The listing builds one solid part. Answer for the finished solid, in the listing's coordinates (mm). A direction names the side the tool comes from. Coordinates: 2 decimals unless noted, no trailing zeros. Order: outer loops, then holes, each group sorted by start corner. A loop starts at its lowest first (then second) coordinate and runs counter-clockwise, first axis right, second up. Notation, with made-up numbers: (-21.75, 21.5) - (34.25, 21.5) arc R14 ccw to (34.25, 30.5) - close; hole circle Ø4 at (36.5, 16.5). An arc over 180 degrees is marked (long way). Use a Markdown table: item, result. Add a question column.
Item 1: Find the intervals of material crossed by line 1 along X through (y, z) = (0, 11); line 2 along X through (y, z) = (21, -12); line 3 along Z through (x, y) = (17.25, -6), in increasing order.
Item 2: The part is cut by section A-A, the plane z = 0. Give the vertices of the cut face in (x, y), then the cut area to 3 significant figures.
Item 3: The part is cut by section B-B, the plane x = 13.5. Give the vertices of the cut face in (y, z), then the cut area to 3 significant figures.
Item 4: Flat-ended cylindrical pins translate along their axes: P1, Ø1.5, axis at x = 12.5, z = 0.5, coming from the -Y side; P2, Ø1.2, axis at x = 9.5, z = 0.5, coming from the +Y side; P3, Ø2, axis at x = 10.5, y = -6.5, coming from the +Z side. Find the tip coordinate at first contact, or state that the pin passes through.
Item 5: The part is cut by section D-D, the plane x = 6. Give the vertices of the cut face in (y, z), then the cut area to 3 significant figures.
Item 6: For faces 1 (the cylindrical face through (11, 0, 13)), 2 (the cylindrical face through (11, 13, 0)), 3 (the flat face through (9, -7, 2)), 4 (the cylindrical face through (11.59, -0.88, -19.98)), determine the directions among +Z, -Z, +X, -X, +Y, -Y from which every point of the face is accessible in a straight line to the end or side of a thin tool.
Item 7: The part is cut by section C-C, the plane y = -1.5. Give the vertices of the cut face in (x, z).
Item 8: The mould has two halves that part along Z. Classify faces 5 (the flat face through (5, 20.2, 1.9)), 6 (the flat face through (9, -8.1, 0)), 7 (the cylindrical face through (2.535, -18.518, -20.195)): released by +Z, released by -Z, zero draft, split by the parting line, or undercut.
from build123d import *

# Parameters (mm, degrees)
SKETCH_2_R               = 6
CUT_EXTRUDE_1_DEPTH      = 45.55917414
HOLE_WIZARD_M6_1_REACH   = 58.389
HOLE_WIZARD_M6_1_BORE_R  = 2.5
PATTERN_CIRCULAR_1_COUNT = 2
PATTERN_CIRCULAR_1_ANGLE = 90
CUT_EXTRUDE_2_REACH      = 46.559
SKETCH_4_W               = 4
SKETCH_4_H               = 4.2
SKETCH_5_R               = 20
CUT_EXTRUDE_3_DEPTH      = 4


with BuildPart() as part:
    # 草图1 → 旋转1 (revolve)
    with BuildSketch(Plane.XY, mode=Mode.PRIVATE) as revolve_1_sk:
        Polygon((0, 0), (0, 27.4), (5, 27.4), (5, 20), (22, 20), (22, 0), align=None)
    revolve(revolve_1_sk.sketch.rotate(Axis((0, 0, 0), (1, 0, 0)), 90), axis=Axis((0, 0, 0), (1, 0, 0)))

    # 草图2 → 切除-拉伸1 (cut, through all)
    with BuildSketch(Plane.ZY):
        Circle(SKETCH_2_R)
    extrude(amount=-CUT_EXTRUDE_1_DEPTH, mode=Mode.SUBTRACT)

    # M6 螺纹孔1 bore (on position points) → M6 螺纹孔1 (cut, up to next)
    with BuildSketch(Plane(origin=(13.5, 0, 20), x_dir=(1, 0, 0), z_dir=(0, 0, 1)), mode=Mode.PRIVATE) as hole_wizard_m6_1_sk1:
        Circle(HOLE_WIZARD_M6_1_BORE_R)
    hole_wizard_m6_1_tool1 = extrude(hole_wizard_m6_1_sk1.sketch, amount=-HOLE_WIZARD_M6_1_REACH, mode=Mode.PRIVATE) & part.part
    hole_wizard_m6_1 = hole_wizard_m6_1_tool1.solids().sort_by_distance((13.5, 0, 20))[0]
    add(hole_wizard_m6_1, mode=Mode.SUBTRACT)

    # 阵列(圆周)1: M6 螺纹孔1 ×2 about axis
    pattern_circular_1_axis = Axis((22, 0, 0), (-1, 0, 0))
    for i in range(1, PATTERN_CIRCULAR_1_COUNT):
        add(hole_wizard_m6_1.rotate(pattern_circular_1_axis, i * PATTERN_CIRCULAR_1_ANGLE / (PATTERN_CIRCULAR_1_COUNT - 1)), mode=Mode.SUBTRACT)

    # 草图4 → 切除-拉伸2 (cut, up to next)
    with BuildSketch(Plane.ZY, mode=Mode.PRIVATE) as cut_extrude_2_sk1:
        with Locations((0, -6)):
            Rectangle(SKETCH_4_W, SKETCH_4_H)
    cut_extrude_2_tool1 = extrude(cut_extrude_2_sk1.sketch, amount=-CUT_EXTRUDE_2_REACH, mode=Mode.PRIVATE) & part.part
    add(cut_extrude_2_tool1.solids().sort_by_distance((0, -6, 0))[0], mode=Mode.SUBTRACT)

    # 草图5 → 切除-拉伸3 (cut)
    with BuildSketch(Plane(origin=(22, 0, 0), x_dir=(0, 0, -1), z_dir=(1, 0, 0))):
        with Locations(Location((0, 0, 0), (0, 0, 180))):
            Circle(SKETCH_5_R)
    extrude(amount=-CUT_EXTRUDE_3_DEPTH, mode=Mode.SUBTRACT)


solid = part.part
Solution:
| question | item | result |
|---|---|---|
| 1 | line 1 | x = 0 to 11, 16 to 18 |
| 1 | line 2 | x = 0 to 5 |
| 1 | line 3 | z = -19.08 to -2, 2 to 19.08 |
| 2 | outline | (0, -27.4) - (5, -27.4) - (5, -20) - (18, -20) - (18, -8.1) - (0, -8.1) - close; (0, 6) - (11, 6) - (11, 20) - (5, 20) - (5, 27.4) - (0, 27.4) - close; (16, 6) - (18, 6) - (18, 20) - (16, 20) - close |
| 2 | area | 470 mm2 |
| 3 | outline | (-8.1, -2) - (-8.1, 2) - (-5.66, 2) arc R6 cw to (-2.5, 5.45) - (-2.5, 19.84) arc R20 ccw (long way) to (19.84, -2.5) - (5.45, -2.5) arc R6 cw to (-5.66, -2) - close; (2.5, 5.45) arc R6 cw to (5.45, 2.5) - (19.84, 2.5) arc R20 ccw to (2.5, 19.84) - close |
| 3 | area | 993 mm2 |
| 4 | P1 | stops at y = -20 |
| 4 | P2 | stops at y = 20 |
| 4 | P3 | stops at z = 19.23 |
| 5 | outline | circle Ø40 at (0, 0); hole (-8.1, -2) - (-5.66, -2) arc R6 ccw (long way) to (-5.66, 2) - (-8.1, 2) - close |
| 5 | area | 1,130 mm2 |
| 6 | face 1 | +Z |
| 6 | face 2 | +Y |
| 6 | face 3 | +X, -X |
| 6 | face 4 | +X |
| 7 | outline | (0, -27.36) - (5, -27.36) - (5, -19.94) - (18, -19.94) - (18, -5.81) - (0, -5.81) - close; (0, 5.81) - (11.5, 5.81) - (11.5, 19.94) - (5, 19.94) - (5, 27.36) - (0, 27.36) - close; (15.5, 5.81) - (18, 5.81) - (18, 19.94) - (15.5, 19.94) - close |
| 8 | face 5 | zero draft |
| 8 | face 6 | undercut |
| 8 | face 7 | split by the parting line |
